Solid Edge part; units mm, degrees
sketch "Sketch1" plane through (0, 0, 0) normal (0, -1, 0) x (1, 0, 0)
  line L0 (46.2892, 8.8157) -> (46.4009, 6.4567)
  line L1 (46.4009, 6.4567) -> (48.1612, 5.7905)
  line L2 (48.1612, 5.7905) -> (49.8066, 7.4845)
  line L3 (49.8066, 7.4845) -> (50.8439, 6.7003)
  line L4 (50.8439, 6.7003) -> (49.6626, 4.6555)
  line L5 (49.6626, 4.6555) -> (50.7833, 3.1434)
  line L6 (50.7833, 3.1434) -> (53.0833, 3.679)
  line L7 (53.0833, 3.679) -> (53.5319, 2.4584)
  line L8 (53.5319, 2.4584) -> (51.4326, 1.3769)
  line L9 (51.4326, 1.3769) -> (51.5579, -0.5011)
  line L10 (51.5579, -0.5011) -> (53.7824, -1.2941)
  line L11 (53.7824, -1.2941) -> (53.4999, -2.5634)
  line L12 (53.4999, -2.5634) -> (51.1491, -2.3382)
  line L13 (51.1491, -2.3382) -> (50.2393, -3.9858)
  line L14 (50.2393, -3.9858) -> (51.6818, -5.8556)
  line L15 (51.6818, -5.8556) -> (50.7579, -6.7706)
  line L16 (50.7579, -6.7706) -> (48.9022, -5.3101)
  line L17 (48.9022, -5.3101) -> (47.2459, -6.2045)
  line L18 (47.2459, -6.2045) -> (47.4486, -8.5573)
  line L19 (47.4486, -8.5573) -> (46.1767, -8.8276)
  line L20 (46.1767, -8.8276) -> (45.4049, -6.5958)
  line L21 (45.4049, -6.5958) -> (43.5283, -6.4526)
  line L22 (43.5283, -6.4526) -> (42.4267, -8.5415)
  line L23 (42.4267, -8.5415) -> (41.2106, -8.0813)
  line L24 (41.2106, -8.0813) -> (41.768, -5.7865)
  line L25 (41.768, -5.7865) -> (40.2667, -4.6514)
  line L26 (40.2667, -4.6514) -> (38.2107, -5.8132)
  line L27 (38.2107, -5.8132) -> (37.4364, -4.7685)
  line L28 (37.4364, -4.7685) -> (39.1459, -3.1393)
  line L29 (39.1459, -3.1393) -> (38.4966, -1.3728)
  line L30 (38.4966, -1.3728) -> (36.1389, -1.2386)
  line L31 (36.1389, -1.2386) -> (36.0523, 0.0589)
  line L32 (36.0523, 0.0589) -> (38.3713, 0.5052)
  line L33 (38.3713, 0.5052) -> (38.7801, 2.3423)
  line L34 (38.7801, 2.3423) -> (36.8691, 3.73)
  line L35 (36.8691, 3.73) -> (37.498, 4.8685)
  line L36 (37.498, 4.8685) -> (39.6899, 3.99)
  line L37 (39.6899, 3.99) -> (41.0271, 5.3145)
  line L38 (41.0271, 5.3145) -> (40.1697, 7.5148)
  line L39 (40.1697, 7.5148) -> (41.314, 8.1329)
  line L40 (41.314, 8.1329) -> (42.683, 6.2081)
  line L41 (42.683, 6.2081) -> (44.5236, 6.5998)
  line L42 (44.5236, 6.5998) -> (44.9926, 8.9145)
  line L43 (44.9926, 8.9145) -> (46.2892, 8.8157)
  circle A0 centre (44.9678, 0.0085) radius 2.5
extrude "Protrusion1" add sketch "Sketch1" against normal blind 9
sketch "Sketch2" plane through (44.9173, 9, 0.0434) normal (0, 1, 0) x (-0.9971, 0, 0.076)
  circle A0 centre (-0.053, -0.031) radius 10.5
  circle A1 centre (-0.053, -0.031) radius 2.5
extrude "ExtrudedProtrusion_2" add sketch "Sketch2" along normal blind 6.5
sketch "Sketch3" plane through (44.9678, 15.5, 0.0085) normal (0, 1, 0) x (0, 0, 1)
  line L0 (-3.1085, 7.5) -> (3.0915, 7.5)
  line L1 (3.0915, 7.5) -> (3.0915, 5)
  line L2 (3.0915, 5) -> (-3.1085, 5)
  line L3 (-3.1085, 5) -> (-3.1085, 7.5)
  dimension "D1" = 3.1085
  dimension "D2" = 3.1085
extrude "ExtrudedCutout_1" cut sketch "Sketch3" against normal blind 6
sketch "Sketch4" plane through (49.9678, 12.8, 0) normal (1, 0, 0) x (0, -1, 0)
  line L0 (3.3, -3.1) -> (3.3, -1.6566)
  line L1 (3.3, -1.6566) -> (0.8, -3.1)
  line L2 (0.8, -3.1) -> (3.3, -3.1)
  line L3 (0.8, 3.1) -> (3.3, 1.6566)
  line L4 (3.3, 1.6566) -> (3.3, 3.1)
  line L5 (3.3, 3.1) -> (0.8, 3.1)
extrude "Protrusion2" add sketch "Sketch4" along normal up to vertex (2.5 mm away)
sketch "Sketch5" plane through (49.9678, 12.7, 0) normal (1, 0, 0) x (0, 0, 1)
  circle A0 centre (0, 0.275) radius 1.7
extrude "Cutout1" cut sketch "Sketch5" against normal up to vertex (5 mm away) and the other way up to vertex (5.5 mm away)
sketch "Sketch6" plane through (44.9678, 15.5, 0.0085) normal (0, 1, 0) x (1, 0, 0)
  line L0 (3.3967, 3.7849) -> (1.5, 3.7849)
  line L1 (1.5, 3.7849) -> (1.5, -3.5131)
  line L2 (1.5, -3.5131) -> (3.3967, -3.5131)
  line L3 (3.3967, -3.5131) -> (3.3967, 3.7849)
  line L4 (-3.7072, 3.8625) -> (-1.5, 3.8625)
  line L5 (-1.5, 3.8625) -> (-1.5, -3.5519)
  line L6 (-1.5, -3.5519) -> (-3.7072, -3.5519)
  line L7 (-3.7072, -3.5519) -> (-3.7072, 3.8625)
extrude "Protrusion3" add sketch "Sketch6" against normal up to vertex (15.5 mm away)
Model file for the job. Use its own axes, mm. A direction names the side the tool comes from. Give positions to 0.01 mm unless a question says otherwise; leave off trailing zeros. Write each loop counter-clockwise with the first axis right and the second up, starting at its lowest first coordinate (ties: lowest second). Pieces come first, ordered by that corner, then holes. Notation, with made-up numbers: (81, 20) - (104, 20) arc R7 cw to (104, 30) - close; hole circle Ø3 at (-6.5, 5.5). An arc over 180 degrees is marked (long way). One line per question, with ' | ' between items. Start each with the question number.
(1) 3-axis set-ups, long thin cutter, end or side, ignore diameter. For faces 1 (the face through (38.279, 4.437, -3.965)), 2 (the face through (44.95, 12.2, -2.49)), 3 (the face through (48.972, 4.437, 6.626)): which of +Z, -Z, +X, -X, +Y, -Y reach the whole face in a straight line?
(2) Two-plate mould, pull along X, no slides. Class faces 4 (the face through (34.742, 12.204, -2.375)), 5 (the face through (52.341, 4.437, -2.452)), 6 (the face through (51.494, 4.437, 0.451)): +X half, -X half, draft (parallel to the pull), parting line (faces both ways), or undercut.
(3) Slice it at D-D on y = 13.5. Write the cut outline in (x, z), plus the area to 3 significant figures.
(4) Slice it at A-A on y = 11. Write the cut outline in (x, z).
(5) Slice it at C-C on z = -3.5. Write the cut outline in (x, y).
(6) Slice it at B-B on x = 40.75. Write the cut outline in (y, z), plus the area to 3 significant figures.
(7) Wall check: line 1 along Y through (x, z) = (54.3, 0) (3 decimals); line 2 along Y through (x, z) = (49.05, 0) (3 decimals); line 3 along X through (y, z) = (14.5, -2.25). Give the ranges that are in metal, low to high. Write a range as from..to.
(8) Pin check, flat tips, straight feed: P1, Ø3, axis at x = 51.5, z = -0.5, coming from the +Y side; P2, Ø6, axis at y = 2.5, z = 3.5, coming from the +X side; P3, Ø2.5, axis at y = 12.425, z = 0, coming from the +X side; P4, Ø1.5, axis at y = 4.5, z = -3.5, coming from the +X side. Stop position of each tip, or through.
Results below:
1) face 1: -X, -Y | face 2: +Y, -Y | face 3: +Z, -Y
2) face 4: parting line | face 5: undercut | face 6: +X half
3) outline: (48.36, -1.32) - (48.36, 1.32) - (49.97, 1.32) - (49.97, 3.1) - (52.47, 3.1) - (52.47, 1.32) - (55.39, 1.32) arc R10.5 ccw (long way) to (55.38, -1.32) - (52.47, -1.32) - (52.47, -3.1) - (49.97, -3.1) - (49.97, -1.32) - close; hole (43.47, -1.99) arc R2.5 ccw to (46.47, -1.99) - (46.47, 2.01) arc R2.5 ccw to (43.47, 2.01) - close | area: 305 mm^2
4) outline: (48.36, -0.93) - (48.36, 0.93) - (49.97, 0.93) - (49.97, 2.52) - (52.47, 2.52) - (52.47, 0.93) - (55.43, 0.93) arc R10.5 ccw (long way) to (55.43, -0.93) - (52.47, -0.93) - (52.47, -2.52) - (49.97, -2.52) - (49.97, -0.93) - close; hole (43.47, -1.99) arc R2.5 ccw to (46.47, -1.99) - (46.47, 2.01) arc R2.5 ccw to (43.47, 2.01) - close
5) outline: (35.07, 9) - (38.77, 9) - (38.77, 0) - (50.51, 0) - (50.51, 9) - (54.86, 9) - (54.86, 15.5) - (35.07, 15.5) - close
6) outline: (0, -5.02) - (9, -5.02) - (9, -9.61) - (15.5, -9.61) - (15.5, 9.62) - (9, 9.62) - (9, 7.83) - (0, 7.83) - (0, 6.03) - (9, 6.03) - (9, 5.04) - (0, 5.04) - close | area: 232 mm^2
7) line 1: 9..10.725, 14.125..15.5 | line 2: 0..10.725, 14.125..15.5 | line 3: 34.71..43.9, 46.04..49.97, 52.47..55.22
8) P1: y = 15.5 | P2: x = 53.53 | P3: x = 48.36 | P4: x = 50.92
